Read the model definition and answer for the solid it produces. Units are mm, in the model's axes. Coordinates: 2 decimals unless noted, no trailing zeros. Order: outer loops, then holes, each group sorted by start corner. A loop starts at its lowest first (then second) coordinate and runs counter-clockwise, first axis right, second up.
Autodesk Inventor part; units mm, degrees
ref_plane "YZ Plane" through (0, 0, 0) normal (1, 0, 0) x (0, 1, 0)
ref_plane "XZ Plane" through (0, 0, 0) normal (0, 1, 0) x (-1, 0, 0)
ref_plane "XY Plane" through (0, 0, 0) normal (0, 0, 1) x (1, 0, 0)
sketch "Sketch1" plane through (0, 0, 0) normal (0, 1, 0) x (-1, 0, 0)
  line L0 (-21, 29) -> (21, 29)
  line L1 (21, 29) -> (21, -29)
  line L2 (21, -29) -> (-21, -29)
  line L3 (-21, -29) -> (-21, 29)
  line L4 (-21, 29) -> (21, -29) construction
  line L5 (21, 29) -> (-21, -29) construction
  point P0 (0, 0)
  dimension "d0" = 42
  dimension "d1" = 58
extrude "Extrusion1" add sketch "Sketch1" along normal blind 1
sketch "Sketch2" plane through (0, 1, 0) normal (0, 1, 0) x (1, 0, 0)
  line L0 (-20.998, 28.8101) -> (20.8952, 28.8101) construction
  line L1 (20.8952, 28.8101) -> (20.8952, -28.9985) construction
  line L2 (20.8952, -28.9985) -> (-20.998, -28.9985) construction
  line L3 (-20.998, -28.9985) -> (-20.998, 28.8101) construction
  point P0 (0, 0)
sketch "Sketch3" plane through (0, 0, 0) normal (0, -1, 0) x (1, 0, 0)
  line L0 (-20.9976, 28.7529) -> (21.0508, 28.7529) construction
  line L1 (21.0508, 28.7529) -> (21.0508, -28.9972) construction
  line L2 (21.0508, -28.9972) -> (-20.9976, -28.9972) construction
  line L3 (-20.9976, -28.9972) -> (-20.9976, 28.7529) construction
  point P0 (0, 0)
sketch "Sketch4" plane through (0, 0, 0) normal (0, -1, 0) x (1, 0, 0)
  line L0 (-21, 29) -> (21, 29)
  line L1 (21, 29) -> (18.5, 29)
  line L2 (18.5, 29) -> (18.5, 26.5)
  line L3 (18.5, 26.5) -> (21, 26.5)
  line L4 (21, 26.5) -> (21, 29)
  circle A0 centre (18.5, 26.5) radius 1.25
  point P0 (0, 0)
  dimension "d42" = 2.5
  dimension "d43" = 2.5
  dimension "d44" = 2.5
extrude "Extrusion2" cut sketch "Sketch4" against normal through all contours A0 L3 L2 | L2 L3 A0
sketch "Sketch5" plane through (0, 0, 0) normal (0, -1, 0) x (1, 0, 0)
  line L0 (-21, -29) -> (21, -29)
  line L1 (-21, -29) -> (-18.5, -29)
  line L2 (-18.5, -29) -> (-18.5, -26.5)
  line L3 (-18.5, -26.5) -> (-21, -26.5)
  line L4 (-21, -26.5) -> (-21, -29)
  circle A0 centre (-18.5, -26.5) radius 1.25
  point P0 (0, 0)
  dimension "d49" = 2.5
  dimension "d50" = 2.5
  dimension "d51" = 2.5
extrude "Extrusion3" cut sketch "Sketch5" against normal through all contours A0 L3 L2 | L2 L3 A0
sketch "Sketch6" plane through (0, 1, 0) normal (0, 1, 0) x (1, 0, 0)
  line L0 (-21, -29) -> (21, -29)
  line L1 (-21, -29) -> (-18.5, -29)
  line L2 (-18.5, -29) -> (-18.5, -26.5)
  line L3 (-18.5, -26.5) -> (-21, -26.5)
  line L4 (-21, -26.5) -> (-21, -29)
  circle A0 centre (-18.5, -26.5) radius 1.25
  point P0 (0, 0)
  dimension "d60" = 2.5
  dimension "d61" = 2.5
  dimension "d62" = 2.5
extrude "Extrusion4" cut sketch "Sketch6" against normal up to next contours A0 L3 L2 | L2 L3 A0
properties part number "regulator"
1) Straight lines are drawn through the part: line 1 (Z direction, x = -18.5, y = 0.4); line 2 (Z direction, x = 18.5, y = 0.7); line 3 (X direction, y = 0.65, z = 27). For each, find the intervals that lie inside material, in ascending order.
A:
line 1: z = -29 to -27.75, -25.25 to 25.25, 27.75 to 29
line 2: z = -29 to 25.25, 27.75 to 29
line 3: x = -21 to -19.65, -17.35 to 17.35, 19.65 to 21
2) A cutting plane is placed at B-B, the plane z = -26.5. Determine the outline of the cut face in (x, y), and give its area (3 significant figures).
A:
outline: (-21, 0) - (-19.75, 0) - (-19.75, 1) - (-21, 1) - close; (-17.25, 0) - (21, 0) - (21, 1) - (-17.25, 1) - close
area: 39.5 mm2
3) A cutting plane is placed at D-D, the plane z = 26.5. Determine the outline of the cut face in (x, y), and give its area (3 significant figures).
A:
outline: (-21, 0) - (-19.75, 0) - (-19.75, 1) - (-21, 1) - close; (-17.25, 0) - (17.25, 0) - (17.25, 1) - (-17.25, 1) - close; (19.75, 0) - (21, 0) - (21, 1) - (19.75, 1) - close
area: 37.0 mm2
4) Determine the mould class of faces 1 (the cylindrical face through (-17.345, 0.493, -26.979)), 2 (the flat face through (0, 0, 0)) for opening direction X: pulls with the +X half, pulls with the -X half, needs draft (parallel to the pull), parting line crosses it, or undercut.
A:
face 1: undercut
face 2: needs draft
5) A cutting plane is placed at C-C, the plane x = -18.5. Determine the outline of the cut face in (y, z), and give its area (3 significant figures).
A:
outline: (0, -29) - (1, -29) - (1, -27.75) - (0, -27.75) - close; (0, -25.25) - (1, -25.25) - (1, 25.25) - (0, 25.25) - close; (0, 27.75) - (1, 27.75) - (1, 29) - (0, 29) - close
area: 53.0 mm2
6) A cutting plane is placed at A-A, the plane x = 18.5. Determine the outline of the cut face in (y, z).
A:
outline: (0, -29) - (1, -29) - (1, 25.25) - (0, 25.25) - close; (0, 27.75) - (1, 27.75) - (1, 29) - (0, 29) - close
7) A flat-ended cylindrical pin translates along its axis: pin 1 Ø2 at (x, z) = (-18.5, -26.5) entering from -Y. Find the tip coordinate at first contact, or state that the pin passes through.
A:
pin 1: passes through
